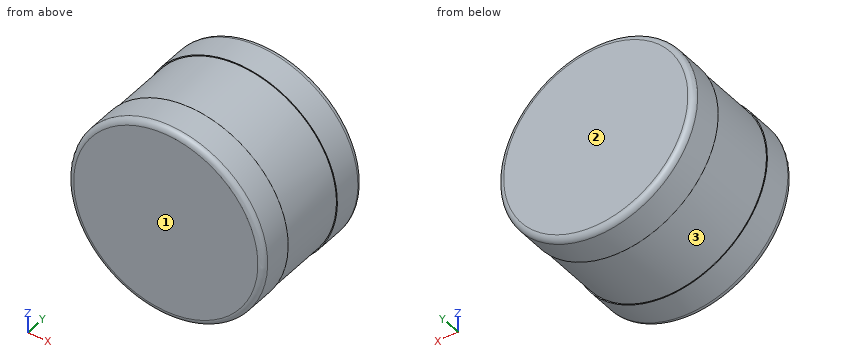
from build123d import *

# Parameters (mm, degrees)
SKETCH_1_R      = 51.5
EXTRUDE_1_DEPTH = 72
FILLET_1_R      = 3


with BuildPart() as part:
    # 草图1 → 凸台-拉伸1 (new body)
    with BuildSketch(Plane(origin=(0, 0, 0), x_dir=(1, 0, 0), z_dir=(0, 1, 0))):
        with Locations(Location((0, 0, 0), (0, 0, 270))):
            Circle(SKETCH_1_R)
    extrude(amount=EXTRUDE_1_DEPTH)

    # 圆角1
    fillet_1_edges = [part.edges().sort_by_distance(p)[0] for p in [
        (0, 0, -51.5),
        (0, 72, -51.5),
    ]]
    fillet(fillet_1_edges, radius=FILLET_1_R)

    # 草图2 → 切除-旋转1 (revolve, cut)
    with BuildSketch(Plane.XY, mode=Mode.PRIVATE) as cut_revolve_1_sk:
        Polygon((51.5, 36), (51.5, 54), (51, 54), (51, 18), (51.5, 18), align=None)
    revolve(cut_revolve_1_sk.sketch.rotate(Axis((0, 0, 0), (0, 1, 0)), 90), axis=Axis((0, 0, 0), (0, 1, 0)), mode=Mode.SUBTRACT)


solid = part.part
Geometry: final body of the model. Coordinates: model frame, mm. Face numbers are marked on the shaded views. Give positions to 0.01 mm unless a question says otherwise; leave off trailing zeros. Loops run counter-clockwise (first coordinate to the right, second up) from the corner with the lowest first, then second, coordinate; pieces in that order, holes last. Notation, with made-up numbers: (8, 11) - (61, 11) arc R21 ccw to (61, 17) - close; hole circle Ø4 at (31.25, -9.5). An arc over 180 degrees is marked (long way). Answer as CSV lines item,"result". Start each with the question number.
1. Pin query (flat end, axial travel): P1, Ø12, axis at y = 41.5, z = -3.5, coming from the -X side; P2, Ø5, axis at y = 28, z = -5.5, coming from the -X side; P3, Ø2, axis at x = -29.5, y = 43, coming from the +Z side; P4, Ø3, axis at x = 23, z = 27.5, coming from the -Y side. Return the tip coordinate at first contact, or that it passes through.
2. Draft query along Y for the marked faces 1, 2 and 3. Return one class per face: released by +Y, released by -Y, zero draft, split by the parting line, or undercut.
3. Section A-A, the plane y = 60. Return loops of the section in (x, z), plus the area to 3 significant figures.
4. Ray query, L1, parallel to Z at x = -40, y = 45.5; L2, parallel to Z at x = 45.5, y = 17.5; L3, parallel to X at y = 66.5, z = 9. Return the intervals inside material, ascending.
Answers:
1,P1,"stops at x = -51"
1,P2,"stops at x = -50.91"
1,P3,"stops at z = 42.29"
1,P4,"stops at y = 0"
2,face 1,"released by -Y"
2,face 2,"released by +Y"
2,face 3,"undercut"
3,outline,"circle Ø103 at (0, 0)"
3,area,"8,330 mm2"
4,L1,"z = -31.64 to 31.64"
4,L2,"z = -24.12 to 24.12"
4,L3,"x = -50.71 to 50.71"
